Autodesk Inventor part; units mm, degrees
ref_plane "YZ Plane" through (0, 0, 0) normal (1, 0, 0) x (0, 1, 0)
ref_plane "XZ Plane" through (0, 0, 0) normal (0, 1, 0) x (-1, 0, 0)
ref_plane "XY Plane" through (0, 0, 0) normal (0, 0, 1) x (1, 0, 0)
sketch "Sketch1" plane through (0, 0, 0) normal (0, 0, 1) x (1, 0, 0)
  line L0 (-27.5, 50) -> (27.5, 50)
  line L1 (27.5, 50) -> (27.5, -50)
  line L2 (27.5, -50) -> (-27.5, -50)
  line L3 (-27.5, -50) -> (-27.5, 50)
  point P0 (0, 0)
  point P1 (0, 50)
  dimension "d0" = 50
  dimension "d2" = 100
  dimension "d3" = 55
  dimension "d4" = 27.5
extrude "Extrusion1" add sketch "Sketch1" along normal blind 3
sketch "Sketch2" plane through (-27.5, -50, 0) normal (0, -1, 0) x (1, 0, 0)
  line L0 (31.45, 0) -> (23.55, 0)
  line L1 (23.55, 0) -> (23.55, 3)
  line L2 (23.55, 3) -> (31.45, 3)
  line L3 (31.45, 3) -> (31.45, 0)
  line L4 (31.45, 0) -> (23.55, 3) construction
  line L5 (23.55, 0) -> (31.45, 3) construction
  line L6 (0, 0) -> (55, 0)
  line L7 (0, 3) -> (55, 3)
  line L8 (55, 0) -> (55, 3)
  line L9 (0, 0) -> (0, 3)
  point P0 (27.5, 0)
  point P1 (27.5, 1.5)
  point P2 (55, 1.5)
  point P3 (31.45, 1.5)
  point P4 (0, 1.5)
  point P5 (27.5, 0)
  dimension "d8" = 7.9
extrude "Extrusion2" add sketch "Sketch2" along normal blind 12.1 contours L0 L1 L2 L3
properties part number "AcrylicPane"
Could you check a few things on this model? Use its own coordinates, in mm. A direction names the side the tool comes from. Give positions to 0.01 mm unless a question says otherwise; leave off trailing zeros. Order: outer loops, then holes, each group sorted by start corner. A loop starts at its lowest first (then second) coordinate and runs counter-clockwise, first axis right, second up.
1. Suppose I cut it at B-B (x = -17.5). List the corners of the cut face in (y, z) for me.
2. For faces 1 (the flat face through (3.95, -56, 2)), 2 (the flat face through (0, -5, 0)), 3 (the flat face through (-3.95, -56, 1)), which set-ups out of +Z, -Z, +X, -X, +Y, -Y let a thin tool reach every point of the face, with its end or its side?
3. Will these pins go through, and if not, where does the flat tip stop? P1, Ø12, axis at x = -17.5, y = -44.5, coming from the -Z side; P2, Ø1.5, axis at x = 13.5, z = 1, coming from the -Y side; P3, Ø0.9, axis at y = -57, z = 1, coming from the -X side.
4. I need wall thicknesses on L1, parallel to Y at x = 12, z = 2.85. Which ranges of the line are inside material? Lowest first, please.
5. Suppose I cut it at A-A (z = 1.2). List the corners of the cut face in (x, y) for me.
Solved:
1. outline: (-50, 0) - (50, 0) - (50, 3) - (-50, 3) - close
2. face 1: +Z, -Z, +X, -Y
2. face 2: -Z, +X, -X, +Y, -Y
2. face 3: +Z, -Z, -X, -Y
3. P1: stops at z = 0
3. P2: stops at y = -50
3. P3: stops at x = -3.95
4. L1: y = -50 to 50
5. outline: (-27.5, -50) - (-3.95, -50) - (-3.95, -62.1) - (3.95, -62.1) - (3.95, -50) - (27.5, -50) - (27.5, 50) - (-27.5, 50) - close
